from build123d import *

# Parameters (mm, degrees)
F0_R     = 28.575
F0_R_2   = 26.67
F1_DEPTH = 101.6
F2_R     = 28.575
F3_DEPTH = 3.175
F5_DEPTH = 98.425


with BuildPart() as f1:
    # F0 (on Top) → F1 (new body)
    with BuildSketch(Plane.XY):
        Circle(F0_R)
        Circle(F0_R_2, mode=Mode.SUBTRACT)
    extrude(amount=F1_DEPTH)

    # F2 (on face) → F3 (join)
    with BuildSketch(Plane.XY.offset(101.6)):
        Polygon((-17.0136255064, 34.7249471966), (-34.1751240194, 18.0927142501), (-38.2828867267, -5.4503205912), (-27.7678878919, -26.9115182162), (-6.6464996782, -38.0934305715), (17.0136255064, -34.7249471966), (34.1751240194, -18.0927142501), (38.2828867267, 5.4503205912), (27.7678878919, 26.9115182162), (6.6464996782, 38.0934305715), align=None)
        Circle(F2_R, mode=Mode.SUBTRACT)
    extrude(amount=-F3_DEPTH)

    # F4 (on face) → F5 (cut)
    with BuildSketch(Plane(origin=(0, 0, 0), x_dir=(1, 0, 0), z_dir=(0, 0, -1))):
        with BuildLine():
            Line((16.5036009964, -23.3272754336), (15.546752443, -21.669965124))
            ThreePointArc((15.546752443, -21.669965124), (13.335, -23.0968975189), (10.993364075, -24.298865124))
            Line((10.993364075, -24.298865124), (11.9502126283, -25.9561754336))
            ThreePointArc((11.9502126283, -25.9561754336), (14.2875, -24.7466759131), (16.5036009964, -23.3272754336))
        make_face()
        with BuildLine():
            ThreePointArc((10.993364075, 24.298865124), (13.335, 23.0968975189), (15.546752443, 21.669965124))
            Line((15.546752443, 21.669965124), (16.5036009964, 23.3272754336))
            ThreePointArc((16.5036009964, 23.3272754336), (14.2875, 24.7466759131), (11.9502126283, 25.9561754336))
            Line((11.9502126283, 25.9561754336), (10.993364075, 24.298865124))
        make_face()
        with BuildLine():
            Line((-28.4538136247, -2.6289), (-26.540116518, -2.6289))
            ThreePointArc((-26.540116518, -2.6289), (-26.67, 0), (-26.540116518, 2.6289))
            Line((-26.540116518, 2.6289), (-28.4538136247, 2.6289))
            ThreePointArc((-28.4538136247, 2.6289), (-28.575, 0), (-28.4538136247, -2.6289))
        make_face()
    extrude(amount=-F5_DEPTH, mode=Mode.SUBTRACT)


solid = f1.part
Build history of the part. All positions in model axes, mm. A direction names the side the tool comes from. Give positions to 0.01 mm unless a question says otherwise; leave off trailing zeros. Write each loop counter-clockwise with the first axis right and the second up, starting at its lowest first coordinate (ties: lowest second). Pieces come first, ordered by that corner, then holes. Notation, with made-up numbers: (63, -22) - (112, -22) arc R15 ccw to (112, -11) - close; hole circle Ø3 at (16, 60). An arc over 180 degrees is marked (long way). Use one line per item in the form item = value. Start each with the question number.
1. Drop flat-ended pins along their axis: pin 1 Ø5 at (y, z) = (-4.5, 80) entering from -X; pin 2 Ø12 at (x, y) = (26, -5) entering from +Z; pin 3 Ø3 at (x, z) = (-25, 32.5) entering from -Y; pin 4 Ø12 at (y, z) = (-26.5, 29.5) entering from -X. Give the stop position or say it passes through.
2. Band-saw the part on B-B on x = -15.5. Write the cut outline in (y, z) (3 decimals).
3. Band-saw the part on C-C on y = 0. Write the cut outline in (x, z) (3 decimals).
4. Band-saw the part on A-A on z = 91.5. Write the cut outline in (x, y) (3 decimals), plus the area to 3 significant figures.
5. Two-plate mould, pull along Y, no slides. Class faces 1 (the face through (-5.782, -26.036, 50.089)), 2 (the face through (17.4, 32.4, 100)), 3 (the face through (-14, 23, 0)): released by +Y, released by -Y, zero draft, split by the parting line, or undercut.
6. Band-saw the part on D-D on x = 0. Write the cut outline in (y, z) (3 decimals), plus the area to 3 significant figures.
7. Probe line 1 (Y direction, x = 0, z = 70) (3 decimals); line 2 (X direction, y = -17.5, z = 58.5); line 3 (Y direction, x = 24, z = 53). List the from-to ranges inside material, lowest first. Write a range as [from, to].
8. 3-axis set-ups, long thin cutter, end or side, ignore diameter. For faces 4 (the face through (-14.62, -24.55, 48.52)), 5 (the face through (-13.955, 24.935, 48.524)), 6 (the face through (28.572, -0.382, 48.524)), 7 (the face through (-17.4, -32.4, 100)): which of +Z, -Z, +X, -X, +Y, -Y reach the whole face in a straight line?
Conclusion:
q1.pin_1 = -28.45
q1.pin_2 = 101.6
q1.pin_3 = -16.26
q1.pin_4 = -19.91
q2.outline = (-33.406, 98.425) - (-24.006, 98.425) - (-24.006, 0) - (-21.703, 0) - (-21.703, 101.6) - (-33.406, 101.6) - close; (21.703, 0) - (24.006, 0) - (24.006, 98.425) - (34.94, 98.425) - (34.94, 101.6) - (21.703, 101.6) - close
q3.outline = (-37.332, 98.425) - (-26.67, 98.425) - (-26.67, 101.6) - (-37.332, 101.6) - close; (26.67, 0) - (28.575, 0) - (28.575, 98.425) - (37.332, 98.425) - (37.332, 101.6) - (26.67, 101.6) - close
q4.outline = (-28.454, -2.629) arc R28.575 ccw to (11.95, -25.956) - (10.993, -24.299) arc R26.67 cw to (-26.54, -2.629) - close; (-28.454, 2.629) - (-26.54, 2.629) arc R26.67 cw to (10.993, 24.299) - (11.95, 25.956) arc R28.575 ccw to start; (15.547, -21.67) - (16.504, -23.327) arc R28.575 ccw to (16.504, 23.327) - (15.547, 21.67) arc R26.67 cw to start
q4.area = 301 mm²
q5.face_1 = undercut
q5.face_2 = released by +Y
q5.face_3 = zero draft
q6.outline = (-37.147, 98.425) - (-28.575, 98.425) - (-28.575, 0) - (-26.67, 0) - (-26.67, 101.6) - (-37.147, 101.6) - close; (26.67, 0) - (28.575, 0) - (28.575, 98.425) - (37.147, 98.425) - (37.147, 101.6) - (26.67, 101.6) - close
q6.area = 442 mm²
q7.line_1 = [-28.575, -26.67], [26.67, 28.575]
q7.line_2 = [-22.59, -20.13], [20.13, 22.59]
q7.line_3 = [-15.51, -11.63], [11.63, 15.51]
q8.face_4 = -Z, -Y
q8.face_5 = -Z, +Y
q8.face_6 = -Z, +X
q8.face_7 = +Z, -Z, -X, -Y
